```python
from build123d import *

# Parameters (mm, degrees)
SKETCH_1_W      = 57
SKETCH_1_H      = 46
SKETCH_1_R      = 11
SKETCH_1_R_2    = 1.6
EXTRUDE_1_DEPTH = 8
SKETCH_2_W      = 20
SKETCH_2_H      = 40
EXTRUDE_2_DEPTH = 200
SKETCH_3_W      = 51
SKETCH_3_H      = 46
SKETCH_3_R      = 4
EXTRUDE_3_DEPTH = 8


with BuildPart() as part:
    # 草图1 → 凸台-拉伸1 (new body)
    with BuildSketch(Plane.XY):
        Rectangle(SKETCH_1_W, SKETCH_1_H)
        with Locations((-7.5, 0)):
            Circle(SKETCH_1_R, mode=Mode.SUBTRACT)
        with Locations((-23, 15.5)):
            Circle(SKETCH_1_R_2, mode=Mode.SUBTRACT)
        with Locations((8, 15.5)):
            Circle(SKETCH_1_R_2, mode=Mode.SUBTRACT)
        with Locations((8, -15.5)):
            Circle(SKETCH_1_R_2, mode=Mode.SUBTRACT)
        with Locations((-23, -15.5)):
            Circle(SKETCH_1_R_2, mode=Mode.SUBTRACT)
    extrude(amount=EXTRUDE_1_DEPTH)

    # 草图2 → 凸台-拉伸2 (add)
    with BuildSketch(Plane.XY.offset(8)):
        with Locations((18.5, 0)):
            Rectangle(SKETCH_2_W, SKETCH_2_H)
    extrude(amount=EXTRUDE_2_DEPTH)

    # 草图3 → 凸台-拉伸3 (add)
    with BuildSketch(Plane.XY.offset(208)):
        with Locations((3, 0)):
            Rectangle(SKETCH_3_W, SKETCH_3_H)
        with Locations((-7.5, 0)):
            Circle(SKETCH_3_R, mode=Mode.SUBTRACT)
    extrude(amount=EXTRUDE_3_DEPTH)


solid = part.part
```
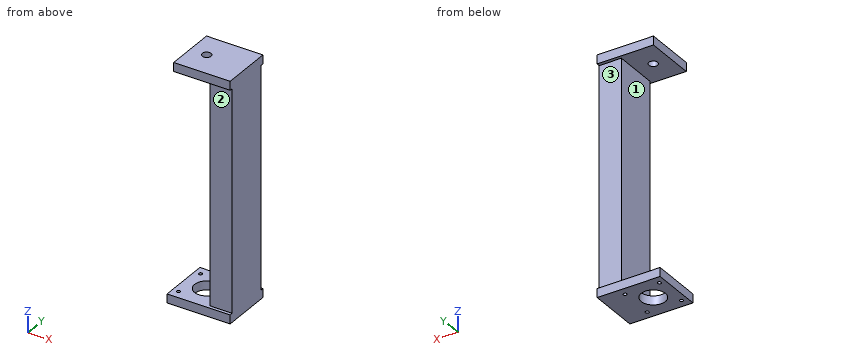
For this review, take the finished solid that the model builds, in its own axes (mm). Face numbers are marked on the shaded views. A direction names the side the tool comes from. Round coordinates to 2 decimals unless told otherwise and drop trailing zeros. Loops run counter-clockwise (first coordinate to the right, second up) from the corner with the lowest first, then second, coordinate; pieces in that order, holes last.
(1) We need section A-A (x = -7.5). Give the boundary of the cut face in (y, z), plus the area to 3 significant figures.
Returned:
outline: (-23, 0) - (-11, 0) - (-11, 8) - (-23, 8) - close; (-23, 208) - (-4, 208) - (-4, 216) - (-23, 216) - close; (4, 208) - (23, 208) - (23, 216) - (4, 216) - close; (11, 0) - (23, 0) - (23, 8) - (11, 8) - close
area: 496 mm2
(2) We need section B-B (z = 30). Give the boundary of the cut face in (x, y).
Returned:
outline: (8.5, -20) - (28.5, -20) - (28.5, 20) - (8.5, 20) - close
(3) Tool access review of the marked faces 1, 2 and 3: name each direction out of +Z, -Z, +X, -X, +Y, -Y from which nothing blocks a thin tool from reaching the whole face with its end or side.
Returned:
face 1: -X, +Y, -Y
face 2: +X, -X, -Y
face 3: +X, -X, +Y
(4) Wall thickness on line 1 along Y through (x, z) = (8, 4); line 2 along Z through (x, y) = (-12, 18); line 3 along X through (y, z) = (-15, 5): over which ranges is each line inside the solid? List them lowest first.
Returned:
line 1: y = -23 to -17.1, -13.9 to 13.9, 17.1 to 23
line 2: z = 0 to 8, 208 to 216
line 3: x = -28.5 to -24.52, -21.48 to 6.48, 9.52 to 28.5
(5) Clearance check with flat-ended pins moving along their axes: P1, Ø0.9, axis at x = 9, y = -16, coming from the -Z side; P2, Ø9, axis at x = -7.5, y = 0, coming from the -Z side; P3, Ø6, axis at x = 16.5, z = 127, coming from the -Y side. State where each tip first meets the part, or that it passes through.
Returned:
P1: stops at z = 8
P2: stops at z = 208
P3: stops at y = -20
(6) We need section C-C (x = 1). Give the boundary of the cut face in (y, z).
Returned:
outline: (-23, 0) - (-6.98, 0) - (-6.98, 8) - (-23, 8) - close; (-23, 208) - (23, 208) - (23, 216) - (-23, 216) - close; (6.98, 0) - (23, 0) - (23, 8) - (6.98, 8) - close
